Geometry check sheet. Reference: the model listing, model coordinates, mm. Face numbers are marked on the shaded views. A direction names the side the tool comes from. Give positions to 0.01 mm unless a question says otherwise; leave off trailing zeros. Loops run counter-clockwise (first coordinate to the right, second up) from the corner with the lowest first, then second, coordinate; pieces in that order, holes last.
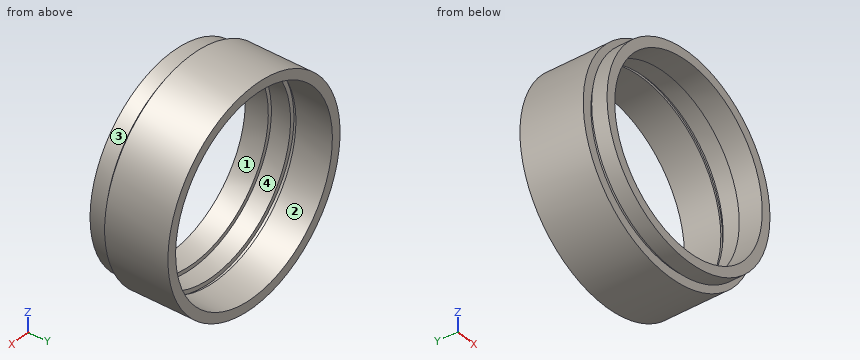
```python
from build123d import *


with BuildPart() as part:
    # 草图1 → 旋转1 (revolve)
    with BuildSketch(Plane.XY, mode=Mode.PRIVATE) as revolve_1_sk:
        Polygon((24, 0), (26.5, 0), (26.5, 4), (25.5, 4), (25.5, 5), (28, 5), (28, 21.5), (25.5, 21.5), (25.5, 12), (26.1, 12), (26.1, 11), (25, 11), (25, 6), (24, 6), align=None)
    revolve(revolve_1_sk.sketch.rotate(Axis((0, 0, 0), (0, 1, 0)), 90), axis=Axis((0, 0, 0), (0, 1, 0)))  # turned: the seam where the file's is


solid = part.part
```
1) Depth check by flat-ended pin: P1, Ø5, axis at y = 17, z = 18, coming from the +X side; P2, Ø4, axis at y = 19.5, z = 20.5, coming from the +X side; P3, Ø12, axis at x = 5, z = -17, coming from the +Y side; P4, Ø2, axis at x = 14, y = 6, coming from the -Z side. Enter the tip coordinate at first touch or a pass-through.
2) Sectioned sample at A-A on x = 0. Enter the section's corners in (y, z).
3) Tool access check on the marked faces 1 and 2. Record the directions out of +Z, -Z, +X, -X, +Y, -Y that give a thin tool (end or side, any length) a straight path to the whole face; none if there is none.
4) Sectioned sample at B-B on z = 0. Enter the section's corners in (x, y), plus the area to 3 significant figures.
5) Scan lines: line 1 along X through (y, z) = (9.85, 0); line 2 along Z through (x, y) = (13.5, 9); line 3 along Z through (x, y) = (-4, 17.5). Record each from-to range of solid material in increasing order.
6) Sectioned sample at C-C on y = 17. Enter the section's corners in (x, z), plus the area to 3 significant figures.
7) Sectioned sample at D-D on y = 10.25. Enter the section's corners in (x, z), plus the area to 3 significant figures.
8) Mould release check, pull along Z, two halves, no side actions. Record for the marked faces 3 and 4: +Z half, -Z half, draft (parallel to the pull), parting line (faces both ways), or undercut.
Determined:
1. P1: stops at x = 23.32
1. P2: stops at x = 21.02
1. P3: passes through
1. P4: stops at z = -24.8
2. outline: (0, -26.5) - (4, -26.5) - (4, -25.5) - (5, -25.5) - (5, -28) - (21.5, -28) - (21.5, -25.5) - (12, -25.5) - (12, -26.1) - (11, -26.1) - (11, -25) - (6, -25) - (6, -24) - (0, -24) - close; (0, 24) - (6, 24) - (6, 25) - (11, 25) - (11, 26.1) - (12, 26.1) - (12, 25.5) - (21.5, 25.5) - (21.5, 28) - (5, 28) - (5, 25.5) - (4, 25.5) - (4, 26.5) - (0, 26.5) - close
3. face 1: +Y, -Y
3. face 2: +Y
4. outline: (-28, 5) - (-25.5, 5) - (-25.5, 4) - (-26.5, 4) - (-26.5, 0) - (-24, 0) - (-24, 6) - (-25, 6) - (-25, 11) - (-26.1, 11) - (-26.1, 12) - (-25.5, 12) - (-25.5, 21.5) - (-28, 21.5) - close; (24, 0) - (26.5, 0) - (26.5, 4) - (25.5, 4) - (25.5, 5) - (28, 5) - (28, 21.5) - (25.5, 21.5) - (25.5, 12) - (26.1, 12) - (26.1, 11) - (25, 11) - (25, 6) - (24, 6) - close
4. area: 112 mm2
5. line 1: x = -28 to -25, 25 to 28
5. line 2: z = -24.53 to -21.04, 21.04 to 24.53
5. line 3: z = -27.71 to -25.18, 25.18 to 27.71
6. outline: circle Ø56 at (0, 0); hole circle Ø51 at (0, 0)
6. area: 420 mm2
7. outline: circle Ø56 at (0, 0); hole circle Ø50 at (0, 0)
7. area: 500 mm2
8. face 3: parting line
8. face 4: undercut
